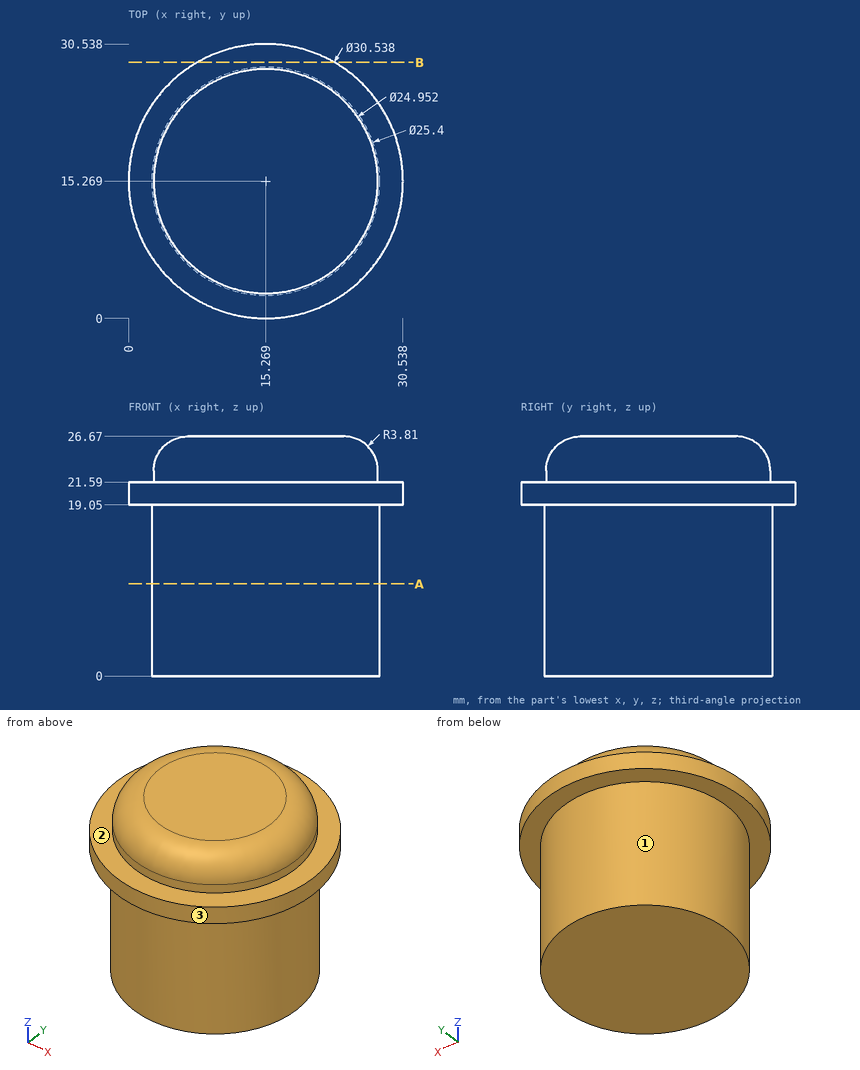
Study the drawing (mm; zero at the part's minimum x, y, z) and answer. A direction names the side the tool comes from. Round coordinates to 2 decimals unless told otherwise and drop trailing zeros. Write each loop counter-clockwise with the first axis right and the second up, starting at its lowest first coordinate (ties: lowest second). Pieces come first, ordered by that corner, then holes.
1) Straight lines are drawn through the part: line 1 (Z direction, x = 3.5, y = 20.5); line 2 (X direction, y = 15, z = 2.75); line 3 (X direction, y = 13.5, z = 18) (1 decimal). For each, find the intervals that lie inside material, in ascending order.
2) A tool of negligible diameter and unlimited length cuts with its end or side. For the marked faces 1, 2 and 3, from which of +Z, -Z, +X, -X, +Y, -Y can it reach the whole face along a straight path? Write none if from no direction.
3) A cutting plane is placed at A-A (z = 10.25). Give the vertices of the cut face in (x, y), plus the area to 3 significant figures.
4) Given pin 1 Ø8 at (x, z) = (5, 22.5) entering from -Y; pin 2 Ø12 at (x, y) = (4, 9.5) entering from +Z; pin 3 Ø2 at (x, z) = (6, 23.5) entering from -Y; pin 4 Ø6 at (y, z) = (22, 13) entering from +X, each flat-ended and moving along its own axis, determine where each tip first touches the part or whether it passes through.
5) A cutting plane is placed at B-B (y = 28.5). Give the vertices of the cut face in (x, z), plus the area to 3 significant figures.
Completed:
1. line 1: z = 19.05 to 21.59
1. line 2: x = 2.57 to 27.97
1. line 3: x = 2.7 to 27.8
2. face 1: -Z
2. face 2: +Z
2. face 3: +Z, -Z
3. outline: circle Ø25.4 at (15.27, 15.27)
3. area: 507 mm2
4. pin 1: stops at y = 1.39
4. pin 2: stops at z = 26.67
4. pin 3: stops at y = 5.98
4. pin 4: stops at x = 27.41
5. outline: (7.65, 19.05) - (22.89, 19.05) - (22.89, 21.59) - (7.65, 21.59) - close
5. area: 38.7 mm2
